Can you work these out from the model? Positions are in its coordinate system, mm. A direction names the side the tool comes from. Give positions to 0.01 mm unless a question says otherwise; leave off trailing zeros. Order: outer loops, then holes, each group sorted by start corner. A loop starts at its lowest first (then second) coordinate and runs counter-clockwise, first axis right, second up. Notation, with made-up numbers: M 31,-24.75 L 57,-24.75 A29 ccw 57,-4.75 Z; hole C 87.25,53.25 d6. An arc over 180 degrees is marked long. Answer as a JSON object with one key per item and string values.
```python
from build123d import *

# Parameters (mm, degrees)
F2_R = 9.5
F4_R = 2


# Not quite as in the source:
# - a fillet or chamfer that OpenCascade refuses, or shapes differently, is made with other operations: its cross-section is extruded or revolved along the edge and cut away or added


with BuildPart() as f1:
    # F0 (on Front) → F1 (revolve)
    with BuildSketch(Plane.XZ):
        Polygon((0, 4.25), (0, 0), (64, 0), (64, 9.5), (8, 9.5), (8, 4.25), align=None)
    revolve(axis=Axis((32, 0, 0), (1, 0, 0)))

    # F2
    f2_edges = [f1.edges().sort_by_distance(p)[0] for p in [
        (64, 0, -9.5),
    ]]
    fillet(f2_edges, radius=F2_R)

    # F3: fillet of radius 9 on 1 edges, made by hand

    # F3_s1 → F3_t2 (revolve, cut)
    with BuildSketch(Plane.XZ):
        with BuildLine():
            ThreePointArc((16.181534086, 9.5), (11.3209785622, 8.0746287038), (8, 4.25))
            Line((8, 4.25), (8, 9.5))
            Line((8, 9.5), (16.181534086, 9.5))
        make_face()
    revolve(axis=Axis((8, 0, 0), (1, 0, 0)), mode=Mode.SUBTRACT)

    # F4
    f4_edges = [f1.edges().sort_by_distance(p)[0] for p in [
        (0, 0, -4.25),
    ]]
    fillet(f4_edges, radius=F4_R)


solid = f1.part
```
1) For faces 1 (the face through (4.958, -3.584, 2.285)), 2 (the face through (35.07, 8.43, 4.38)), which set-ups out of +Z, -Z, +X, -X, +Y, -Y let a thin tool reach every point of the face, with its end or its side?
Results found:
{"face 1": "-X", "face 2": "+X, -X"}
2) I'm going to push flat-ended pins straight in: pin 1 Ø4 at (y, z) = (5, 1) entering from +X; pin 2 Ø6 at (x, z) = (11, 4) entering from -Y; pin 3 Ø6 at (x, y) = (34.5, -5.5) entering from +Z. Where does each tip first touch, or does it pass through?
Results found:
{"pin 1": "stops at x = 63.48", "pin 2": "stops at y = -8.79", "pin 3": "stops at z = 9.17"}
3) I want a section at A-A on x = 25.5. Write out the boundary of the cut face in (y, z), and give its area (3 significant figures).
Results found:
{"outline": "C 0,0 d19", "area": "284 mm²"}
4) I need wall thicknesses on L1, parallel to Y at x = 25.5, z = -8.5; L2, parallel to Y at x = 32, z = 0.5. Which ranges of each line are inside material? Lowest first, please.
Results found:
{"L1": "y = -4.24 to 4.24", "L2": "y = -9.49 to 9.49"}
